```python
from build123d import *

# Parameters (mm, degrees)
SKETCH1_R           = 2.0701
BOSS_EXTRUDE1_DEPTH = 2.286


with BuildPart() as part:
    # Sketch1 → Boss-Extrude1 (new body)
    with BuildSketch(Plane.XY.offset(2.286)):
        with BuildLine():
            Line((41.2908279, 38.357320472), (-11.4935, 7.88227455))
            Line((-11.4935, 7.88227455), (-12.573, 6.012525703))
            Line((-12.573, 6.012525703), (-12.573, -54.937566141))
            Line((-12.573, -54.937566141), (-12.014209682, -57.023))
            Line((-12.014209682, -57.023), (10.487566141, -57.023))
            Line((10.487566141, -57.023), (12.573, -56.464209682))
            Line((12.573, -56.464209682), (12.573, -10.925199144))
            ThreePointArc((12.573, -10.925199144), (13.423738686, -7.750199144), (15.748, -5.42593783))
            Line((15.748, -5.42593783), (55.185939989, 17.343567439))
            Line((55.185939989, 17.343567439), (54.627149671, 19.429001298))
            Line((54.627149671, 19.429001298), (43.6988795, 38.357320472))
            Line((43.6988795, 38.357320472), (41.2908279, 38.357320472))
        make_face()
        Circle(SKETCH1_R, mode=Mode.SUBTRACT)
        with Locations((0, -38.1)):
            Circle(SKETCH1_R, mode=Mode.SUBTRACT)
        with Locations((0, -12.7)):
            Circle(SKETCH1_R, mode=Mode.SUBTRACT)
        with Locations((0, -25.4)):
            Circle(SKETCH1_R, mode=Mode.SUBTRACT)
        with Locations((0, -50.8)):
            Circle(SKETCH1_R, mode=Mode.SUBTRACT)
        with Locations((32.995567884, 19.05)):
            Circle(SKETCH1_R, mode=Mode.SUBTRACT)
        with Locations((10.998522628, 6.35)):
            Circle(SKETCH1_R, mode=Mode.SUBTRACT)
        with Locations((21.997045256, 12.7)):
            Circle(SKETCH1_R, mode=Mode.SUBTRACT)
        with Locations((43.994090512, 25.4)):
            Circle(SKETCH1_R, mode=Mode.SUBTRACT)
    extrude(amount=-BOSS_EXTRUDE1_DEPTH)


solid = part.part
```
For this review, take the finished solid that the model builds, in its own axes (mm). A direction names the side the tool comes from. Coordinates: 2 decimals unless noted, no trailing zeros. Write each loop counter-clockwise with the first axis right and the second up, starting at its lowest first coordinate (ties: lowest second). Pieces come first, ordered by that corner, then holes.
(1) For pin 1 Ø6.5 at (x, y) = (0, -25.4) entering from +Z; pin 2 Ø0.7 at (y, z) = (-25, 1) entering from +X; pin 3 Ø2.5 at (x, y) = (33, 19.05) entering from -Z, all flat-tipped, find the tip position at first contact; note any pin that passes through.
(2) Add section B-B on z = 1.4. Count the separate pieces of the cut face and the enclosed holes in it, then the cut area to 3 significant figures.
(3) Wall thickness on probe 1 along Y at (x, z) = (0, 1.2); probe 2 along X at (y, z) = (-29, 0.95); probe 3 along X at (y, z) = (-38.5, 0.5): over which ranges is each line inside the solid? List them lowest first.
(4) Tool access review of faces 5 (the face through (12.573, -34, 1)), 6 (the face through (-12.298, -55.966, 1.159)): name each direction out of +Z, -Z, +X, -X, +Y, -Y from which nothing blocks a thin tool from reaching the whole face with its end or side.
(5) Add section C-C on y = 25.4. Give the boundary of the cut face in (x, z).
(6) Add section A-A on y = -50.8. Give the boundary of the cut face in (x, z).
(7) Add section D-D on x = 48. Give the boundary of the cut face in (y, z), then the cut area to 3 significant figures.
(8) The part is to be moulded in two halves that separate along X. For faces 1 (the face through (15.268, 23.333, 1.159)), 2 (the face through (-1, -57.023, 1)), 3 (the face through (30.927, 19.141, 1.159)), 4 (the face through (54.91, 18.37, 1.16)), say which applies: +X half, -X half, draft (parallel to the pull), parting line (faces both ways), or undercut.
Answer sheet:
1. pin 1: stops at z = 2.29
1. pin 2: stops at x = 12.57
1. pin 3: passes through
2. separate pieces: 1
2. enclosed holes: 9
2. area: 2,750 mm2
3. probe 1: y = -57.02 to -52.87, -48.73 to -40.17, -36.03 to -27.47, -23.33 to -14.77, -10.63 to -2.07, 2.07 to 14.52
3. probe 2: x = -12.57 to 12.57
3. probe 3: x = -12.57 to -2.03, 2.03 to 12.57
4. face 5: +Z, -Z, +X, -Y
4. face 6: +Z, -Z, -X, -Y
5. outline: (18.85, 0) - (41.92, 0) - (41.92, 2.29) - (18.85, 2.29) - close; (46.06, 0) - (51.18, 0) - (51.18, 2.29) - (46.06, 2.29) - close
6. outline: (-12.57, 0) - (-2.07, 0) - (-2.07, 2.29) - (-12.57, 2.29) - close; (2.07, 0) - (12.57, 0) - (12.57, 2.29) - (2.07, 2.29) - close
7. outline: (13.19, 0) - (30.91, 0) - (30.91, 2.29) - (13.19, 2.29) - close
7. area: 40.5 mm2
8. face 1: -X half
8. face 2: draft
8. face 3: undercut
8. face 4: +X half
